from build123d import *

# Parameters (mm, degrees)
SKETCH_1_R          = 8.5
EXTRUDE_1_DEPTH     = 30
SKETCH_2_R          = 3.1
EXTRUDE_2_DEPTH     = 1
SKETCH_3_R          = 0.75
EXTRUDE_3_DEPTH     = 5.2
SKETCH_4_R          = 1.05
CUT_EXTRUDE_1_DEPTH = 1


with BuildPart() as part:
    # 草图1 → 凸台-拉伸1 (new body)
    with BuildSketch(Plane(origin=(0, 0, 0), x_dir=(1, 0, 0), z_dir=(0, 1, 0))):
        with Locations(Location((0, 0, 0), (0, 0, 270))):
            Circle(SKETCH_1_R)
    extrude(amount=EXTRUDE_1_DEPTH)

    # 草图2 → 凸台-拉伸2 (add)
    with BuildSketch(Plane(origin=(0, 30, 0), x_dir=(1, 0, 0), z_dir=(0, 1, 0))):
        with Locations(Location((0, 0, 0), (0, 0, 270))):
            Circle(SKETCH_2_R)
    extrude(amount=EXTRUDE_2_DEPTH)

    # 草图3 → 凸台-拉伸3 (add)
    with BuildSketch(Plane(origin=(0, 31, 0), x_dir=(1, 0, 0), z_dir=(0, 1, 0))):
        with Locations(Location((0, 0, 0), (0, 0, 270))):
            Circle(SKETCH_3_R)
    extrude(amount=EXTRUDE_3_DEPTH)

    # 草图4 → 切除-拉伸1 (cut)
    with BuildSketch(Plane(origin=(0, 30, 0), x_dir=(1, 0, 0), z_dir=(0, 1, 0))):
        with Locations(Location((0, 5, 0), (0, 0, 270))):
            Circle(SKETCH_4_R)
        with Locations(Location((4.330127019, 2.5, 0), (0, 0, 270))):
            Circle(SKETCH_4_R)
        with Locations(Location((4.330127019, -2.5, 0), (0, 0, 270))):
            Circle(SKETCH_4_R)
        with Locations(Location((0, -5, 0), (0, 0, 270))):
            Circle(SKETCH_4_R)
        with Locations(Location((-4.330127019, -2.5, 0), (0, 0, 270))):
            Circle(SKETCH_4_R)
        with Locations(Location((-4.330127019, 2.5, 0), (0, 0, 270))):
            Circle(SKETCH_4_R)
    extrude(amount=-CUT_EXTRUDE_1_DEPTH, mode=Mode.SUBTRACT)


solid = part.part
CAD build for the part. Positions are in the model's coordinates, mm. A direction names the side the tool comes from. Round coordinates to 2 decimals unless told otherwise and drop trailing zeros. Write each loop counter-clockwise with the first axis right and the second up, starting at its lowest first coordinate (ties: lowest second). Pieces come first, ordered by that corner, then holes.
(1) 3-axis set-ups, long thin cutter, end or side, ignore diameter. For faces 4 (the face through (8.428, 14.79, -1.107)), 5 (the face through (0, 29, -5)): which of +Z, -Z, +X, -X, +Y, -Y reach the whole face in a straight line?
(2) Slice it at A-A, the plane z = 0. Write the cut outline in (x, y).
(3) Slice it at D-D, the plane z = -2.5. Write the cut outline in (x, y).
(4) Slice it at C-C, the plane y = 18. Write the cut outline in (x, z).
(5) Mould opens along Z. For faces 1 (the face through (0, 36.2, 0)), 2 (the face through (4, 29, 2)), 3 (the face through (0.225, 33.564, 0.715)) say: pulls with the +Z half, pulls with the -Z half, needs draft (parallel to the pull), parting line crosses it, or undercut.
(6) Probe line 1 along X through (y, z) = (29.8, 2.5); line 2 along Y through (x, z) = (-6.5, -0.5); line 3 along X through (y, z) = (29.55, -5). List the from-to ranges inside material, lowest first.
(7) Slice it at B-B, the plane x = 2.25. Write the cut outline in (y, z).
(8) Drop flat-ended pins along their axis: P1, Ø3, axis at x = 1.5, z = -1, coming from the +Y side; P2, Ø2.5, axis at x = 0, z = -5, coming from the +Y side; P3, Ø1.9, axis at x = -4.33, z = 2.5, coming from the +Y side; P4, Ø1.5, axis at y = 9, z = -4.5, coming from the +X side. Give the stop position or say it passes through.
From the geometry:
1. face 4: +Y, -Y
1. face 5: +Y
2. outline: (-8.5, 0) - (8.5, 0) - (8.5, 30) - (3.1, 30) - (3.1, 31) - (0.75, 31) - (0.75, 36.2) - (-0.75, 36.2) - (-0.75, 31) - (-3.1, 31) - (-3.1, 30) - (-8.5, 30) - close
3. outline: (-8.12, 0) - (8.12, 0) - (8.12, 30) - (5.38, 30) - (5.38, 29) - (3.28, 29) - (3.28, 30) - (1.83, 30) - (1.83, 31) - (-1.83, 31) - (-1.83, 30) - (-3.28, 30) - (-3.28, 29) - (-5.38, 29) - (-5.38, 30) - (-8.12, 30) - close
4. outline: circle Ø17 at (0, 0)
5. face 1: needs draft
5. face 2: undercut
5. face 3: parting line crosses it
6. line 1: x = -8.12 to -5.38, -3.28 to 3.28, 5.38 to 8.12
6. line 2: y = 0 to 30
6. line 3: x = -6.87 to -1.05, 1.05 to 6.87
7. outline: (0, -8.2) - (30, -8.2) - (30, -2.13) - (31, -2.13) - (31, 2.13) - (30, 2.13) - (30, 8.2) - (0, 8.2) - close
8. P1: stops at y = 36.2
8. P2: stops at y = 30
8. P3: stops at y = 29
8. P4: stops at x = 7.63
